```python
from build123d import *

# Parameters (mm, degrees)
F0_W     = 88
F0_H     = 5
F1_DEPTH = 5
F2_W     = 23.1
F2_H     = 4
F2_W_2   = 23.2
F3_DEPTH = 17.501
F5_DEPTH = 10.001


# Not quite as in the source:
# - a feature names something its author has since deleted; it is built from what else it names


with BuildPart() as f1:
    # F0 (on Front) → F1 (new body, symmetric)
    with BuildSketch(Plane.XZ):
        Polygon((44, -17.5), (49, -17.5), (49, 17.5), (-49, 17.5), (-49, -17.5), (-44, -17.5), (-44, -12.5), (-44, 9.5), (44, 9.5), (44, -12.5), align=None)
        with Locations((0, -15)):
            Rectangle(F0_W, F0_H)
    extrude(amount=F1_DEPTH, both=True)

    # F2 (on Top) → F3 (cut, through all)
    with BuildSketch(Plane.XY):
        with Locations((-26.7, 0)):
            Rectangle(F2_W, F2_H)
        Rectangle(F2_W, F2_H)
        with Locations((26.75, 0)):
            Rectangle(F2_W_2, F2_H)
    extrude(amount=F3_DEPTH, mode=Mode.SUBTRACT)

    # F4 (on face) → F5 (cut, through all)
    with BuildSketch(Plane.XZ.offset(5)):
        with BuildLine():
            ThreePointArc((-26.7, 15.5), (-28.7, 13.5), (-26.7, 11.5))
            Line((-26.7, 11.5), (-26.7, 15.5))
        make_face()
        with BuildLine():
            Line((-26.7, 15.5), (-26.7, 11.5))
            ThreePointArc((-26.7, 11.5), (-25.2857864376, 12.0857864376), (-24.7, 13.5))
            ThreePointArc((-24.7, 13.5), (-25.2857864376, 14.9142135624), (-26.7, 15.5))
        make_face()
        with BuildLine():
            ThreePointArc((0, 15.5), (-2, 13.5), (0, 11.5))
            Line((0, 11.5), (0, 15.5))
        make_face()
        with BuildLine():
            Line((0, 15.5), (0, 11.5))
            ThreePointArc((0, 11.5), (1.4142135624, 12.0857864376), (2, 13.5))
            ThreePointArc((2, 13.5), (1.4142135624, 14.9142135624), (0, 15.5))
        make_face()
        with BuildLine():
            ThreePointArc((26.75, 15.5), (24.75, 13.5), (26.75, 11.5))
            Line((26.75, 11.5), (26.75, 15.5))
        make_face()
        with BuildLine():
            Line((26.75, 15.5), (26.75, 11.5))
            ThreePointArc((26.75, 11.5), (28.1642135624, 12.0857864376), (28.75, 13.5))
            ThreePointArc((28.75, 13.5), (28.1642135624, 14.9142135624), (26.75, 15.5))
        make_face()
    extrude(amount=-F5_DEPTH, mode=Mode.SUBTRACT)


solid = f1.part
```
Read the model definition and answer for the solid it produces. Units are mm, in the model's axes. A direction names the side the tool comes from. Round coordinates to 2 decimals unless told otherwise and drop trailing zeros. Write each loop counter-clockwise with the first axis right and the second up, starting at its lowest first coordinate (ties: lowest second). Pieces come first, ordered by that corner, then holes. Notation, with made-up numbers: (60.25, 7) -> (98.25, 7) arc R23 cw to (98.25, 24) -> close; hole circle Ø10 at (61, 73.25). An arc over 180 degrees is marked (long way). Answer in a Markdown table with one row per item. Add a question column.
1) Find section B-B, the plane z = 1. Determine the outline of the cut face in (x, y), and give its area (3 significant figures).
2) Find section C-C, the plane x = -16.5. Determine the outline of the cut face in (y, z), and give its area (3 significant figures).
3) Which of the six approach directions +Z, -Z, +X, -X, +Y, -Y give full straight-line access (tool end or side, diameter ignored) to faces 1 (the face through (11.55, 0, 13)), 2 (the face through (-1, 0, -17.5)), 3 (the face through (-44, 0, -2))?
4) Consider line 1 (X direction, y = -0.75, z = 13); line 2 (Z direction, x = 22.5, y = -4); line 3 (X direction, y = -3.25, z = 1). Determine where each line is inside the solid, lowest interval first.
5) Given P1, Ø12, axis at x = 7, z = 2.5, coming from the -Y side, flat-ended and moving along its own axis, determine where the tip first touches the part or whether it passes through.
6) Determine the mould class of faces 4 (the face through (49, 0, 0)), 5 (the face through (0.7, -2.3, 17.5)), 6 (the face through (29, -2, 13)) for opening direction X: pulls with the +X half, pulls with the -X half, needs draft (parallel to the pull), parting line crosses it, or undercut.
7) Find section A-A, the plane y = 0. Determine the outline of the cut face in (x, z), and give its area (3 significant figures).
Findings below:
| question | item | result |
|---|---|---|
| 1 | outline | (-49, -5) -> (-44, -5) -> (-44, 5) -> (-49, 5) -> close; (44, -5) -> (49, -5) -> (49, 5) -> (44, 5) -> close |
| 1 | area | 100 mm² |
| 2 | outline | (-5, -17.5) -> (5, -17.5) -> (5, -12.5) -> (-5, -12.5) -> close; (-5, 9.5) -> (-2, 9.5) -> (-2, 17.5) -> (-5, 17.5) -> close; (2, 9.5) -> (5, 9.5) -> (5, 17.5) -> (2, 17.5) -> close |
| 2 | area | 98.0 mm² |
| 3 | face 1 | +Z |
| 3 | face 2 | -Z, +X, -X, +Y, -Y |
| 3 | face 3 | +Y, -Y |
| 4 | line 1 | -49 to -38.25, -15.15 to -11.55, 11.55 to 15.15, 38.35 to 49 |
| 4 | line 2 | -17.5 to -12.5, 9.5 to 17.5 |
| 4 | line 3 | -49 to -44, 44 to 49 |
| 5 | P1 | through |
| 6 | face 4 | pulls with the +X half |
| 6 | face 5 | needs draft |
| 6 | face 6 | undercut |
| 7 | outline | (-49, -17.5) -> (49, -17.5) -> (49, 17.5) -> (38.35, 17.5) -> (38.35, 9.5) -> (44, 9.5) -> (44, -12.5) -> (-44, -12.5) -> (-44, 9.5) -> (-38.25, 9.5) -> (-38.25, 17.5) -> (-49, 17.5) -> close; (-15.15, 9.5) -> (-11.55, 9.5) -> (-11.55, 17.5) -> (-15.15, 17.5) -> close; (11.55, 9.5) -> (15.15, 9.5) -> (15.15, 17.5) -> (11.55, 17.5) -> close |
| 7 | area | 939 mm² |
